Can you work these out from the model? Positions are in its coordinate system, mm. A direction names the side the tool comes from. Give positions to 0.01 mm unless a question says otherwise; leave off trailing zeros. Write each loop counter-clockwise with the first axis right and the second up, starting at its lowest first coordinate (ties: lowest second). Pieces come first, ordered by that corner, then holes. Notation, with made-up numbers: M -19,-22.5 L 28,-22.5 A36 cw 28,12.5 Z; hole C 6,-32.5 d6. An arc over 180 degrees is marked long. Write each question's results on one line, items separated by ' | '.
Autodesk Fusion 360 part; units mm, degrees
sketch "Sketch1" plane through (0, 0, 0) normal (0, 0, 1) x (1, 0, 0)
  circle A0 centre (-10.1925, 0) radius 2.5
  circle A1 centre (-25.1925, 0) radius 2.5
  circle A2 centre (-25.1925, 0) radius 1.6
  circle A3 centre (-10.1925, 0) radius 1.6
  line L0 (-27.6925, 0) -> (-7.6925, 0)
  line L1 (-7.6925, 0) -> (-7.6925, -6)
  line L2 (-7.6925, -6) -> (-27.6925, -6)
  line L3 (-27.6925, -6) -> (-27.6925, 0)
  line L4 (-27.6925, 0) -> (-22.6925, 0)
  line L5 (-20.6925, 0) -> (-14.6925, 0)
  line L6 (-14.6925, 0) -> (-14.6925, -2.5)
  line L7 (-14.6925, -2.5) -> (-20.6925, -2.5)
  line L8 (-20.6925, -2.5) -> (-20.6925, 0)
  line L9 (-27.6925, 0) -> (-2.5588, 0)
  line L10 (-7.6925, -2.8) -> (-27.6925, -2.8)
  line L11 (-27.6925, -2.8) -> (-27.6925, 0)
  circle A4 centre (-25.1925, 0) radius 1.05
  circle A5 centre (-10.1925, 0) radius 1.05
  dimension "d1" = 5
  dimension "d3" = 5
  dimension "d4" = 15
  dimension "d6" = 3.2
  dimension "d7" = 3.2
  dimension "d10" = 6
  dimension "d11" = 5
  dimension "d13" = 2.5
  dimension "d14" = 2.8
  dimension "d21" = 6
  dimension "d22" = 2.1
  dimension "d23" = 2.1
extrude "Extrude1" add sketch "Sketch1" along normal blind 2.8 contours A0 A3 L0 L9 | A0 A1 L0 L1 L3 L6 L7 L8 L9 L10 L11 | A0 A3 L0 L9 | L1 L2 L3 L10 | A1 A2 L0 L4 L9 | A1 A2 L0 L4 L9
extrude "Extrude2" add sketch "Sketch1" along normal blind 4.32 contours L1 L2 L3 L10
chamfer "Chamfer1" distance 1.5 angle 45 2 edges at (-14.6925, 0, 1.4) (-20.6925, 0, 1.4)
chamfer "Chamfer2" distance 0.8 angle 45 2 edges at (-27.6925, -6, 2.16) (-7.6925, -6, 2.16)
extrude "Extrude3" add sketch "Sketch1" along normal up to surface (2.8 mm away) contours A3 L0 L9 A5 | A3 L0 L9 A5 | A2 L0 L4 L9 A4 | A2 L0 L4 L9 A4
equation "d17 = 2.8 mm + 1.52 mm"
Item 1: I want a section at B-B, the plane y = 1.5. Please give me the cut outline in (x, z).
Geometry says:
outline: M -27.19,0 L -23.19,0 L -23.19,2.8 L -27.19,2.8 Z; M -12.19,0 L -8.19,0 L -8.19,2.8 L -12.19,2.8 Z
Item 2: Thinking about a two-plate mould opening in X: for faces 1 (the face through (-7.692, -3, 2)), 2 (the face through (-18, -2.8, 4)), 3 (the face through (-25.33, -1.04, 1.38)), which applies, +X half, -X half, draft (parallel to the pull), parting line (faces both ways), or undercut?
Geometry says:
face 1: +X half | face 2: draft | face 3: undercut
Item 3: If I drill on line 1 (X direction, y = -1.75, z = 2.55); line 2 (Y direction, x = -25.25, z = 2.3); line 3 (Z direction, x = -15.5, y = -2.75), over which ranges is the centre line in solid material (lowest first)? Write a range as from..to.
Geometry says:
line 1: x = -27.69..-20.69, -14.69..-7.69 | line 2: y = -6..-1.05, 1.05..2.5 | line 3: z = 0..2.8
Item 4: I want a section at D-D, the plane z = 3.1. Please give me the cut outline in (x, y).
Geometry says:
outline: M -27.69,-5.2 L -26.89,-6 L -8.49,-6 L -7.69,-5.2 L -7.69,-2.8 L -27.69,-2.8 Z
Item 5: I'm going to push flat-ended pins straight in: pin 1 (1.6 mm diameter, centred on x = -14.5, y = -0.5, fed in from +Z); pin 2 (0.8 mm diameter, centred on x = -15.5, z = 3.5, fed in from +Y); pin 3 (1.5 mm diameter, centred on x = -11.5, z = 2.5, fed in from +Y). Where does each tip first touch, or does it pass through?
Geometry says:
pin 1: stops at z = 2.8 | pin 2: stops at y = -2.8 | pin 3: stops at y = 2.44
Item 6: I want a section at C-C, the plane x = -10. Please give me the cut outline in (y, z), and give its area (3 significant figures).
Geometry says:
outline: M -6,0 L -1.03,0 L -1.03,2.8 L -2.8,2.8 L -2.8,4.32 L -6,4.32 Z; M 1.03,0 L 2.49,0 L 2.49,2.8 L 1.03,2.8 Z | area: 22.9 mm2
Item 7: I want a section at A-A, the plane z = 1.25. Please give me the cut outline in (x, y), and give its area (3 significant figures).
Geometry says:
outline: M -27.69,-5.2 L -26.89,-6 L -8.49,-6 L -7.69,-5.2 L -7.69,0 A2.5 ccw -12.69,0 L -13.19,0 L -14.69,-1.5 L -14.69,-2.5 L -20.69,-2.5 L -20.69,-1.5 L -22.19,0 L -22.69,0 A2.5 ccw -27.69,0 Z; hole C -25.19,0 d2.1; hole C -10.19,0 d2.1 | area: 115 mm2
Item 8: For faces 4 (the face through (-27.3, -5.59, 2.13)), 5 (the face through (-13, -1, 2.8)), 6 (the face through (-21.43, -0.76, 1.42)), which set-ups out of +Z, -Z, +X, -X, +Y, -Y let a thin tool reach every point of the face, with its end or its side?
Geometry says:
face 4: +Z, -Z, -X, -Y | face 5: +Z, +X, -X, +Y | face 6: +Z, -Z, +Y
